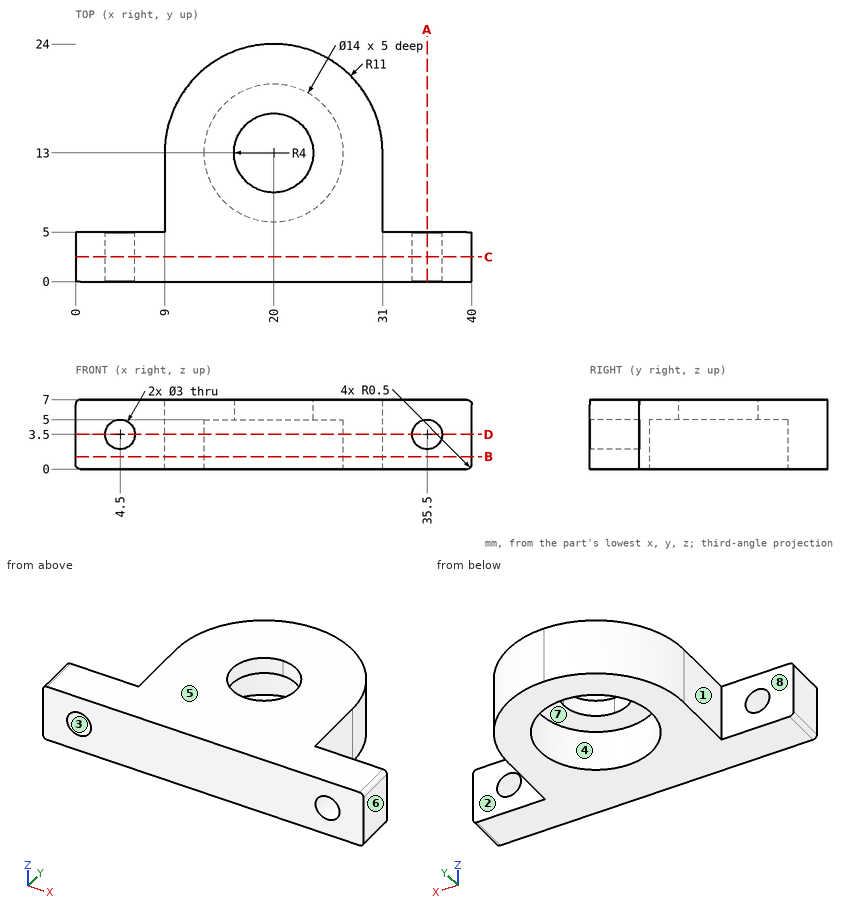
For this review, use the dimensioned drawing (mm, ordinates from the lowest corner) and the shaded views. A direction names the side the tool comes from. Coordinates: 2 decimals unless noted, no trailing zeros. Loops run counter-clockwise (first coordinate to the right, second up) from the corner with the lowest first, then second, coordinate; pieces in that order, holes last. Notation, with made-up numbers: (17, 72.5) - (29, 72.5) arc R21 ccw to (29, 96.5) - close; hole circle Ø3 at (70.5, 29). An arc over 180 degrees is marked (long way). Use one line per item in the form item = value. Start each with the question number.
1) Take a section at C-C (y = 2.5). State the section outline as (x, z) points.
2) For the marked faces 1, 2, 3, 4 and 5, list the 3-axis set-ups (+Z, -Z, +X, -X, +Y, -Y) from which the entire face can be reached by the end or side of a thin tool; tool diameter is ignored.
3) Take a section at A-A (x = 35.5). State the section outline as (y, z) points, plus the area to 3 significant figures.
4) To check wall thickness, follow probe 1 along X at (y, z) = (3.5, 3.5); probe 2 along X at (y, z) = (7.25, 2); probe 3 along X at (y, z) = (3.25, 2.25). State the ranges of each line that lie inside material, in increasing order. Write a range as from..to.
5) Draft analysis for pull direction Y (two halves, no side actions). For the marked faces 6, 7 and 8, state which applies: released by +Y, released by -Y, zero draft, split by the parting line, or undercut.
6) Take a section at B-B (z = 1.25). State the section outline as (x, y) points.
7) Take a section at D-D (z = 3.5). State the section outline as (x, y) points.
8) For pin 1 (11 mm diameter, centred on x = 19, y = 13, fed in from -Z); pin 2 (3 mm diameter, centred on y = 12, z = 3, fed in from +X), all flat-tipped, find the tip position at first contact; note any pin that passes through.
From the geometry:
q1.outline = (0, 0.5) arc R0.5 ccw to (0.5, 0) - (39.5, 0) arc R0.5 ccw to (40, 0.5) - (40, 6.5) arc R0.5 ccw to (39.5, 7) - (0.5, 7) arc R0.5 ccw to (0, 6.5) - close; hole circle Ø3 at (4.5, 3.5); hole circle Ø3 at (35.5, 3.5)
q2.face_1 = +Z, -Z, -X, +Y
q2.face_2 = +Z, -Z, +X, +Y
q2.face_3 = +Y, -Y
q2.face_4 = -Z
q2.face_5 = +Z, +X, -X, +Y, -Y
q3.outline = (0, 0) - (5, 0) - (5, 2) - (0, 2) - close; (0, 5) - (5, 5) - (5, 7) - (0, 7) - close
q3.area = 20.0 mm2
q4.probe_1 = 0..3, 6..34, 37..40
q4.probe_2 = 9..16.01, 23.99..31
q4.probe_3 = 0..3.67, 5.33..34.67, 36.33..40
q5.face_6 = zero draft
q5.face_7 = undercut
q5.face_8 = released by +Y
q6.outline = (0, 0) - (40, 0) - (40, 5) - (31, 5) - (31, 13) arc R11 ccw to (9, 13) - (9, 5) - (0, 5) - close; hole circle Ø14 at (20, 13)
q7.outline = (0, 0) - (3, 0) - (3, 5) - (0, 5) - close; (6, 0) - (34, 0) - (34, 5) - (31, 5) - (31, 13) arc R11 ccw to (9, 13) - (9, 5) - (6, 5) - close; (37, 0) - (40, 0) - (40, 5) - (37, 5) - close; hole circle Ø14 at (20, 13)
q8.pin_1 = 5
q8.pin_2 = 31
